The listing builds one solid part. Answer for the finished solid, in the listing's coordinates (mm). A direction names the side the tool comes from. Give positions to 0.01 mm unless a question says otherwise; leave off trailing zeros. Write each loop counter-clockwise with the first axis right and the second up, starting at its lowest first coordinate (ties: lowest second). Pieces come first, ordered by that corner, then holes. Notation, with made-up numbers: (76, 14.5) - (128, 14.5) arc R26 ccw to (128, 44.5) - close; hole circle Ø8 at (43.25, 50). An arc over 180 degrees is marked (long way). Use a Markdown table: item, result. Add a question column.
from build123d import *

# Parameters (mm, degrees)
PAD_DEPTH       = 5
SKETCH001_R     = 1.8
POCKET_DEPTH    = 5
SKETCH002_R     = 3
POCKET001_DEPTH = 3
SKETCH003_R     = 1.8
POCKET002_DEPTH = 1.8
SKETCH004_R     = 3.7
SKETCH004_R_2   = 2.7
PAD001_DEPTH    = 3
POCKET003_DEPTH = 3


with BuildPart() as part:
    # Sketch → Pad (new body)
    with BuildSketch(Plane.XY):
        Polygon((0, 0), (0, 20), (18, 20), (52, 20), (70, 20), (70, 0), (52, 0), (18, 0), align=None)
    extrude(amount=PAD_DEPTH)

    # Sketch001 → Pocket (cut)
    with BuildSketch(Plane.XY.offset(5)):
        with Locations((5, 15)):
            Circle(SKETCH001_R)
        with Locations((65, 15)):
            Circle(SKETCH001_R)
        with Locations((65, 5)):
            Circle(SKETCH001_R)
        with Locations((5, 5)):
            Circle(SKETCH001_R)
    extrude(amount=-POCKET_DEPTH, mode=Mode.SUBTRACT)

    # Sketch002 → Pocket001 (cut)
    with BuildSketch(Plane.XY.offset(5)):
        with Locations((5, 15)):
            Circle(SKETCH002_R)
        with Locations((65, 15)):
            Circle(SKETCH002_R)
        with Locations((65, 5)):
            Circle(SKETCH002_R)
        with Locations((5, 5)):
            Circle(SKETCH002_R)
    extrude(amount=-POCKET001_DEPTH, mode=Mode.SUBTRACT)

    # Sketch003 → Pocket002 (cut)
    with BuildSketch(Plane.XY.offset(5)):
        with Locations((10, 10)):
            Circle(SKETCH003_R)
        with Locations((20, 10)):
            Circle(SKETCH003_R)
        with Locations((30, 10)):
            Circle(SKETCH003_R)
        with Locations((40, 10)):
            Circle(SKETCH003_R)
        with Locations((50, 10)):
            Circle(SKETCH003_R)
        with Locations((60, 10)):
            Circle(SKETCH003_R)
    extrude(amount=-POCKET002_DEPTH, mode=Mode.SUBTRACT)

    # Sketch004 → Pad001 (new body)
    with BuildSketch(Plane.XY.offset(5)):
        with Locations((10, 10)):
            Circle(SKETCH004_R)
        with Locations((10, 10)):
            Circle(SKETCH004_R_2, mode=Mode.SUBTRACT)
        with Locations((20, 10)):
            Circle(SKETCH004_R)
        with Locations((20, 10)):
            Circle(SKETCH004_R_2, mode=Mode.SUBTRACT)
        with Locations((30, 10)):
            Circle(SKETCH004_R)
        with Locations((30, 10)):
            Circle(SKETCH004_R_2, mode=Mode.SUBTRACT)
        with Locations((40, 10)):
            Circle(SKETCH004_R)
        with Locations((40, 10)):
            Circle(SKETCH004_R_2, mode=Mode.SUBTRACT)
        with Locations((50, 10)):
            Circle(SKETCH004_R)
        with Locations((50, 10)):
            Circle(SKETCH004_R_2, mode=Mode.SUBTRACT)
        with Locations((60, 10)):
            Circle(SKETCH004_R)
        with Locations((60, 10)):
            Circle(SKETCH004_R_2, mode=Mode.SUBTRACT)
    extrude(amount=PAD001_DEPTH)

    # Sketch005 → Pocket003 (cut)
    with BuildSketch(Plane(origin=(0, 0, 0), x_dir=(1, 0, 0), z_dir=(0, 0, -1))):
        Polygon((7, -11.732051), (7, -8.267949), (10, -6.535898), (13, -8.267949), (13, -11.732051), (10, -13.464102), align=None)
        Polygon((17, -11.732051), (17, -8.267949), (20, -6.535898), (23, -8.267949), (23, -11.732051), (20, -13.464102), align=None)
        Polygon((27, -11.732051), (27, -8.267949), (30, -6.535898), (33, -8.267949), (33, -11.732051), (30, -13.464102), align=None)
        Polygon((37, -11.732051), (37, -8.267949), (40, -6.535898), (43, -8.267949), (43, -11.732051), (40, -13.464102), align=None)
        Polygon((47, -11.732051), (47, -8.267949), (50, -6.535898), (53, -8.267949), (53, -11.732051), (50, -13.464102), align=None)
        Polygon((57, -11.732051), (57, -8.267949), (60, -6.535898), (63, -8.267949), (63, -11.732051), (60, -13.464102), align=None)
    extrude(amount=-POCKET003_DEPTH, mode=Mode.SUBTRACT)


solid = part.part
1. Which of the six approach directions +Z, -Z, +X, -X, +Y, -Y give full straight-line access (tool end or side, diameter ignored) to faces 1 (the flat face through (70, 10, 2)), 2 (the cylindrical face through (12.575, 10.811, 6.479)), 3 (the flat face through (43, 10, 1))?
2. The part is cut by section A-A (z = 6). Count the separate pieces of the cut face and the enclosed holes in it, and give its area (3 significant figures).
3. Consider L1, parallel to Y at x = 5, z = 2.5; L2, parallel to Y at x = 5, z = 0.5; L3, parallel to Y at x = 20, z = 3.65. Determine where each line is inside the solid, lowest interval first. Write a range as [from, to].
4. The part is cut by section B-B (x = 5). Give the vertices of the cut face in (y, z), and give its area (3 significant figures).
5. Given P1, Ø5, axis at x = 64.5, y = 14, coming from the +Z side; P2, Ø2, axis at x = 40, y = 10, coming from the +Z side; P3, Ø4, axis at x = 50, y = 10, coming from the +Z side, each flat-ended and moving along its own axis, determine where each tip first touches the part or whether it passes through.
6. The part is cut by section D-D (x = 41). Give the vertices of the cut face in (y, z).
7. For a pull along Y with two mould halves and no side action, classify faces 4 (the cylindrical face through (6.304, 10.163, 6.479)), 5 (the cylindrical face through (9.61, 8.243, 4.113)), 6 (the flat face through (35, 10, 0)) as released by +Y, released by -Y, zero draft, split by the parting line, or undercut.
Check values:
| question | item | result |
|---|---|---|
| 1 | face 1 | +Z, -Z, +X, +Y, -Y |
| 1 | face 2 | +Z |
| 1 | face 3 | -Z |
| 2 | separate pieces | 6 |
| 2 | enclosed holes | 6 |
| 2 | area | 121 mm2 |
| 3 | L1 | y = [0, 2], [8, 12], [18, 20] |
| 3 | L2 | y = [0, 3.2], [6.8, 13.2], [16.8, 20] |
| 3 | L3 | y = [0, 8.2], [11.8, 20] |
| 4 | outline | (0, 0) - (3.2, 0) - (3.2, 2) - (2, 2) - (2, 5) - (0, 5) - close; (6.8, 0) - (13.2, 0) - (13.2, 2) - (12, 2) - (12, 5) - (8, 5) - (8, 2) - (6.8, 2) - close; (16.8, 0) - (20, 0) - (20, 5) - (18, 5) - (18, 2) - (16.8, 2) - close |
| 4 | area | 49.6 mm2 |
| 5 | P1 | stops at z = 8 |
| 5 | P2 | stops at z = 3.2 |
| 5 | P3 | stops at z = 5 |
| 6 | outline | (0, 0) - (7.11, 0) - (7.11, 3) - (12.89, 3) - (12.89, 0) - (20, 0) - (20, 5) - (13.56, 5) - (13.56, 8) - (12.51, 8) - (12.51, 5) - (11.5, 5) - (11.5, 3.2) - (8.5, 3.2) - (8.5, 5) - (7.49, 5) - (7.49, 8) - (6.44, 8) - (6.44, 5) - (0, 5) - close |
| 7 | face 4 | split by the parting line |
| 7 | face 5 | undercut |
| 7 | face 6 | zero draft |
